Geometry check sheet. Reference: the model listing, model coordinates, mm. A direction names the side the tool comes from. Round coordinates to 2 decimals unless told otherwise and drop trailing zeros. Loops run counter-clockwise (first coordinate to the right, second up) from the corner with the lowest first, then second, coordinate; pieces in that order, holes last. Notation, with made-up numbers: M -36,10 L -23,10 A10 ccw -23,17 Z; hole C -2,25 d3. An arc over 180 degrees is marked long. Use one line per item in the form item = value. Start each with the question number.
1. Cross-section at D-D (x = -30). Record the boundary of the cut face in (y, z), then the cut area to 3 significant figures.
2. Cross-section at B-B (x = -46.5). Record the boundary of the cut face in (y, z), then the cut area to 3 significant figures.
3. Material ranges on line 1 (Z direction, x = -19.5, y = 1.75); line 2 (X direction, y = 11.75, z = -7.5); line 3 (X direction, y = 23.25, z = 20.5), recorded low to high.
4. Cross-section at A-A (y = 15). Record the boundary of the cut face in (x, z).
5. Set-up check for faces 1 (the flat face through (-33, 25.4, 6)), 2 (the cylindrical face through (-0.86, 1.5, 10.89)): record each of +Z, -Z, +X, -X, +Y, -Y from which the full face is reachable in a straight line by a thin tool's end or side.
6. Cross-section at C-C (y = 4). Record the boundary of the cut face in (x, z).
7. Go/stop test with flat-tipped pins: pin 1 (4 mm diameter, centred on x = -47.5, y = 14.5, fed in from +Z); pin 2 (10 mm diameter, centred on x = -37.5, y = 10, fed in from +Z); pin 3 (8 mm diameter, centred on x = -36, y = 10, fed in from -Z); pin 4 (12 mm diameter, centred on y = 14.5, z = 21, fed in from +X). Record where each tip stops, or that it passes through.
```python
from build123d import *

# Parameters (mm, degrees)
F1_DEPTH = 25.4
F2_R     = 5


with BuildPart() as f1:
    # F0 (on Front) → F1 (new body)
    with BuildSketch(Plane.XZ):
        with BuildLine():
            ThreePointArc((-40.395132, 36.354515), (-49.048411, 18.696662), (-67.145093, 11.003214))
            Line((-67.145093, 11.003214), (-66.002764, -14.139596))
            Line((-66.002764, -14.139596), (0, -11.140851))
            Line((0, -11.140851), (1.122797, 32.227423))
            Line((1.122797, 32.227423), (-40.395132, 36.354515))
        make_face()
    extrude(amount=-F1_DEPTH)

    # F2
    f2_edges = [f1.edges().sort_by_distance(p)[0] for p in [
        (0.561399, 0, 10.543286),
    ]]
    fillet(f2_edges, radius=F2_R)


solid = f1.part
```
Reported:
q1.outline = M 0,-12.5 L 25.4,-12.5 L 25.4,35.32 L 0,35.32 Z
q1.area = 1,210 mm²
q2.outline = M 0,-13.25 L 25.4,-13.25 L 25.4,21.46 L 0,21.46 Z
q2.area = 882 mm²
q3.line_1 = -12.03 to 34.28
q3.line_2 = -66.3 to 0.09
q3.line_3 = -47.31 to 0.82
q4.outline = M -67.15,11 L -66,-14.14 L 0,-11.14 L 1.12,32.23 L -40.4,36.35 A28.17 cw Z
q5.face_1 = +Z, -Z, +X, -X, +Y
q5.face_2 = -Z, +X, -Y
q6.outline = M -67.15,11 L -66,-14.14 L -0.1,-11.15 L 1.02,32.24 L -40.4,36.35 A28.17 cw Z
q7.pin_1 = 22.77
q7.pin_2 = 36.35
q7.pin_3 = -12.96
q7.pin_4 = 0.99
